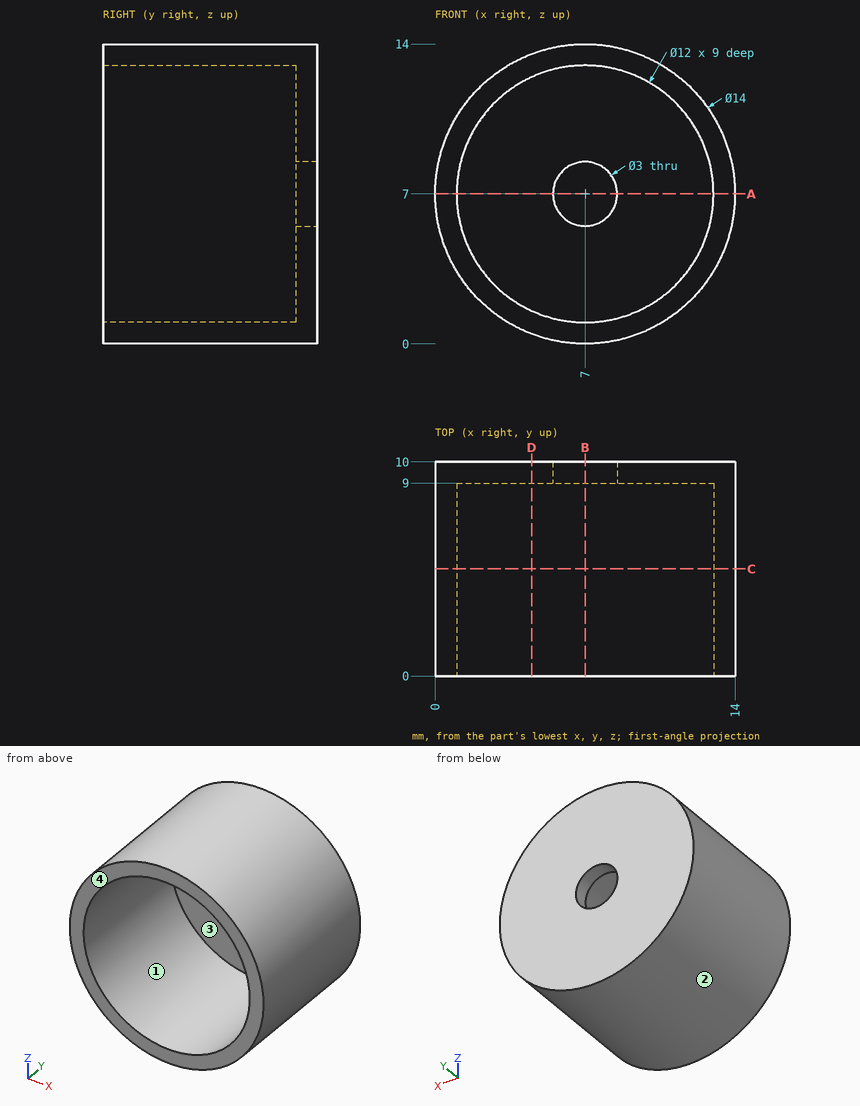
Job drawing, mm, ordinate dimensions from the low corner. One solid piece. Give positions to 0.01 mm unless a question says otherwise; leave off trailing zeros. Write each loop counter-clockwise with the first axis right and the second up, starting at its lowest first coordinate (ties: lowest second). Pieces come first, ordered by that corner, then holes. Notation, with made-up numbers: (4, -34.75) - (27, -34.75) arc R17 ccw to (27, -14.75) - close; hole circle Ø1 at (13.5, -34). An arc over 180 degrees is marked (long way). Answer as CSV lines item,"result".
1. Drill centre lines: L1, parallel to X at y = 9.3, z = 7; L2, parallel to X at y = 1.5, z = 3; L3, parallel to Y at x = 6, z = 10.75. Where is each one in solid material? Low to high. Write a range as [from, to].
Responses:
L1,"x = [0, 5.5], [8.5, 14]"
L2,"x = [1.26, 2.53], [11.47, 12.74]"
L3,"y = [9, 10]"
2. Band-saw the part on D-D (x = 4.5). Write the cut outline in (y, z), and give its area (3 significant figures).
Responses:
outline,"(0, 0.46) - (10, 0.46) - (10, 13.54) - (0, 13.54) - (0, 12.45) - (9, 12.45) - (9, 1.55) - (0, 1.55) - close"
area,"32.6 mm2"
3. Two-plate mould, pull along Z, no slides. Class the marked faces 1, 2, 3 and 4: +Z half, -Z half, draft (parallel to the pull), parting line (faces both ways), or undercut.
Responses:
face 1,"undercut"
face 2,"parting line"
face 3,"undercut"
face 4,"draft"
4. Band-saw the part on C-C (y = 5). Write the cut outline in (x, z), and give its area (3 significant figures).
Responses:
outline,"circle Ø14 at (7, 7); hole circle Ø12 at (7, 7)"
area,"40.8 mm2"
5. Band-saw the part on B-B (x = 7). Write the cut outline in (y, z).
Responses:
outline,"(0, 0) - (10, 0) - (10, 5.5) - (9, 5.5) - (9, 1) - (0, 1) - close; (0, 13) - (9, 13) - (9, 8.5) - (10, 8.5) - (10, 14) - (0, 14) - close"
6. Pin check, flat tips, straight feed: pin 1 (2.5 mm diameter, centred on x = 7, z = 7, fed in from +Y); pin 2 (3 mm diameter, centred on x = 4.5, y = 2.5, fed in from -Z); pin 3 (6 mm diameter, centred on x = 8.5, z = 6, fed in from -Y); pin 4 (2 mm diameter, centred on x = 7.5, y = 4, fed in from +Z). Stop position of each tip, or through.
Responses:
pin 1,"passes through"
pin 2,"stops at z = 0.07"
pin 3,"stops at y = 9"
pin 4,"stops at z = 14"
7. Band-saw the part on A-A (z = 7). Write the cut outline in (x, y), and give its area (3 significant figures).
Responses:
outline,"(0, 0) - (1, 0) - (1, 9) - (5.5, 9) - (5.5, 10) - (0, 10) - close; (8.5, 9) - (13, 9) - (13, 0) - (14, 0) - (14, 10) - (8.5, 10) - close"
area,"29.0 mm2"
